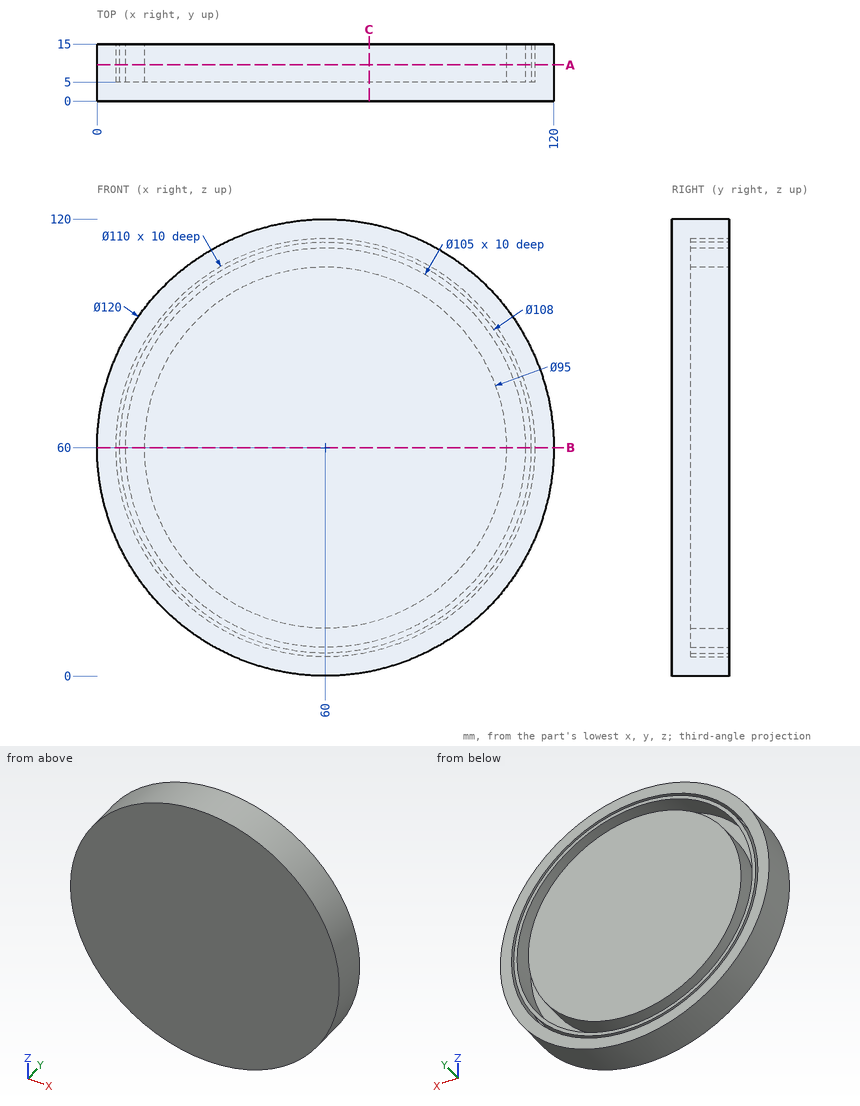
The drawing under review shows one solid part. Ordinate dimensions are in mm from its lowest x, y, z. Coordinates: 2 decimals unless noted, no trailing zeros. Loops run counter-clockwise (first coordinate to the right, second up) from the corner with the lowest first, then second, coordinate; pieces in that order, holes last.
Item 1: Clearance check with flat-ended pins moving along their axes: pin 1 (1.5 mm diameter, centred on y = 5.5, z = 96.5, fed in from +X); pin 2 (6 mm diameter, centred on x = 38.5, z = 50.5, fed in from -Y); pin 3 (4 mm diameter, centred on y = 2.5, z = 24.5, fed in from -X); pin 4 (1.5 mm diameter, centred on y = 2, z = 13, fed in from +X). State where each tip first meets the part, or that it passes through.
Completed:
pin 1: stops at x = 108.19
pin 2: stops at y = 0
pin 3: stops at x = 10.22
pin 4: stops at x = 98.22
Item 2: Add section C-C (x = 71.5). Write out the cut boundary in (y, z) (3 decimals), and give its area (3 significant figures).
Completed:
outline: (0, 1.112) - (15, 1.112) - (15, 6.216) - (5, 6.216) - (5, 7.239) - (15, 7.239) - (15, 8.775) - (5, 8.775) - (5, 13.913) - (15, 13.913) - (15, 106.087) - (5, 106.087) - (5, 111.225) - (15, 111.225) - (15, 112.761) - (5, 112.761) - (5, 113.784) - (15, 113.784) - (15, 118.888) - (0, 118.888) - close
area: 1,640 mm2
Item 3: Add section B-B (z = 60). Write out the cut boundary in (x, y), and give its area (3 significant figures).
Completed:
outline: (0, 0) - (120, 0) - (120, 15) - (115, 15) - (115, 5) - (114, 5) - (114, 15) - (112.5, 15) - (112.5, 5) - (107.5, 5) - (107.5, 15) - (12.5, 15) - (12.5, 5) - (7.5, 5) - (7.5, 15) - (6, 15) - (6, 5) - (5, 5) - (5, 15) - (0, 15) - close
area: 1,680 mm2
Item 4: Wall thickness on L1, parallel to Z at x = 60, y = 12.75; L2, parallel to X at y = 9.25, z = 49.5: over which ranges is each line inside the solid? List them lowest first.
Completed:
L1: z = 0 to 5, 6 to 7.5, 12.5 to 107.5, 112.5 to 114, 115 to 120
L2: x = 0.93 to 6.01, 7.03 to 8.56, 13.68 to 106.32, 111.44 to 112.97, 113.99 to 119.07
Item 5: Add section A-A (y = 9.5). Write out the cut boundary in (x, z), and give its area (3 significant figures).
Completed:
outline: circle Ø120 at (60, 60); circle Ø108 at (60, 60); circle Ø95 at (60, 60); hole circle Ø110 at (60, 60); hole circle Ø105 at (60, 60)
area: 9,400 mm2
